from build123d import *

# Parameters (mm, degrees)
ESQUISSE1_W             = 65.4
ESQUISSE1_H             = 56
BOSS_EXTRU_1_DEPTH      = 1.5
CONG_1_R                = 4
ESQUISSE2_R             = 1.4
ENL_V_MAT_EXTRU_1_DEPTH = 1.5
ESQUISSE3_W             = 12.8
ESQUISSE3_H             = 2.56
BOSS_EXTRU_2_DEPTH      = 2.56
ESQUISSE4_W             = 0.6
ESQUISSE4_H             = 13.16
BOSS_EXTRU_3_DEPTH      = 1.58
ENL_V_MAT_EXTRU_2_REACH = 66.012
ESQUISSE5_W             = 5.9
ESQUISSE5_H             = 0.98
BOSS_EXTRU_4_DEPTH      = 2.56
BOSS_EXTRU_5_DEPTH      = 1.8


with BuildPart() as part:
    # Esquisse1 → Boss.-Extru.1 (new body)
    with BuildSketch(Plane(origin=(0, 0, 0), x_dir=(1, 0, 0), z_dir=(0, 1, 0))):
        Rectangle(ESQUISSE1_W, ESQUISSE1_H)
    extrude(amount=BOSS_EXTRU_1_DEPTH)

    # Congé1
    cong_1_edges = [part.edges().sort_by_distance(p)[0] for p in [
        (32.7, 0.75, 28),
        (-32.7, 0.75, 28),
        (-32.7, 0.75, -28),
        (32.7, 0.75, -28),
    ]]
    fillet(cong_1_edges, radius=CONG_1_R)

    # Esquisse2 → Enlèv. mat.-Extru.1 (cut)
    with BuildSketch(Plane(origin=(0, 1.5, 0), x_dir=(1, 0, 0), z_dir=(0, 1, 0))):
        with Locations(Location((-29, 24.5, 0), (0, 0, 270))):
            Circle(ESQUISSE2_R)
        with Locations(Location((-29, -24.5, 0), (0, 0, 270))):
            Circle(ESQUISSE2_R)
        with Locations(Location((29, -24.5, 0), (0, 0, 270))):
            Circle(ESQUISSE2_R)
        with Locations(Location((29, 24.5, 0), (0, 0, 270))):
            Circle(ESQUISSE2_R)
    extrude(amount=-ENL_V_MAT_EXTRU_1_DEPTH, mode=Mode.SUBTRACT)

    # Esquisse3 → Boss.-Extru.2 (add)
    with BuildSketch(Plane(origin=(0, 1.5, 0), x_dir=(1, 0, 0), z_dir=(0, 1, 0))):
        with Locations((-19.3, 19.72)):
            Rectangle(ESQUISSE3_W, ESQUISSE3_H)
    extrude(amount=BOSS_EXTRU_2_DEPTH)

    # Esquisse4 → Boss.-Extru.3 (add)
    with BuildSketch(Plane(origin=(0, 1.5, 0), x_dir=(1, 0, 0), z_dir=(0, 1, 0))):
        with Locations((-24.42, 20.32)):
            Rectangle(ESQUISSE4_W, ESQUISSE4_H)
        with Locations((-21.86, 20.32)):
            Rectangle(ESQUISSE4_W, ESQUISSE4_H)
        with Locations((-19.3, 20.32)):
            Rectangle(ESQUISSE4_W, ESQUISSE4_H)
        with Locations((-16.74, 20.32)):
            Rectangle(ESQUISSE4_W, ESQUISSE4_H)
        with Locations((-14.18, 20.32)):
            Rectangle(ESQUISSE4_W, ESQUISSE4_H)
    extrude(amount=BOSS_EXTRU_3_DEPTH)

    # Enlèv. mat.-Extru.2: up to this face of the body (flat: up to its plane)
    enl_v_mat_extru_2_end = Plane(part.part.faces().sort_by_distance((-13.88, 2.29, -16.09))[0])
    # Esquisse5 → Enlèv. mat.-Extru.2 (cut, up to the picked face)
    with BuildSketch(Plane.ZY.offset(24.72), mode=Mode.PRIVATE) as enl_v_mat_extru_2_sk1:
        with Locations((-23.95, 1.99)):
            Rectangle(ESQUISSE5_W, ESQUISSE5_H)
    enl_v_mat_extru_2_tool1 = split(extrude(enl_v_mat_extru_2_sk1.sketch, amount=-ENL_V_MAT_EXTRU_2_REACH, mode=Mode.PRIVATE), bisect_by=enl_v_mat_extru_2_end, keep=Keep.BOTH, mode=Mode.PRIVATE)
    # Esquisse5 → Enlèv. mat.-Extru.2 (cut, up to the picked face)
    with BuildSketch(Plane.ZY.offset(24.72), mode=Mode.PRIVATE) as enl_v_mat_extru_2_sk2:
        with BuildLine():
            Line((-17.9329542, 3.08), (-15.267871538, 2.100055504))
            Line((-15.267871538, 2.100055504), (-13.74, 2.100055504))
            ThreePointArc((-13.74, 2.100055504), (-13.106146425, 2.552094428), (-13.327063257, 3.298623259))
            Line((-13.327063257, 3.298623259), (-17.9329542, 3.47707173))
            Line((-17.9329542, 3.47707173), (-17.9329542, 3.08))
        make_face()
    enl_v_mat_extru_2_tool2 = split(extrude(enl_v_mat_extru_2_sk2.sketch, amount=-ENL_V_MAT_EXTRU_2_REACH, mode=Mode.PRIVATE), bisect_by=enl_v_mat_extru_2_end, keep=Keep.BOTH, mode=Mode.PRIVATE)
    # Esquisse5 → Enlèv. mat.-Extru.2 (cut, up to the picked face)
    with BuildSketch(Plane.ZY.offset(24.72), mode=Mode.PRIVATE) as enl_v_mat_extru_2_sk3:
        Polygon((-18.44, 2.48), (-18.039767565, 2.48), (-15.374533954, 1.5), (-18.44, 1.5), align=None)
    enl_v_mat_extru_2_tool3 = split(extrude(enl_v_mat_extru_2_sk3.sketch, amount=-ENL_V_MAT_EXTRU_2_REACH, mode=Mode.PRIVATE), bisect_by=enl_v_mat_extru_2_end, keep=Keep.BOTH, mode=Mode.PRIVATE)
    add(enl_v_mat_extru_2_tool1.solids().sort_by(Axis((-24.72, 1.99, -23.95), (1, 0, 0)))[0], mode=Mode.SUBTRACT)
    add(enl_v_mat_extru_2_tool2.solids().sort_by(Axis((-24.72, 2.834984, -15.224036), (1, 0, 0)))[0], mode=Mode.SUBTRACT)
    add(enl_v_mat_extru_2_tool3.solids().sort_by(Axis((-24.72, 1.864391, -17.402771), (1, 0, 0)))[0], mode=Mode.SUBTRACT)

    # Esquisse6 → Boss.-Extru.4 (add)
    with BuildSketch(Plane(origin=(0, 1.5, 0), x_dir=(1, 0, 0), z_dir=(0, 1, 0))):
        Polygon((-31.5, 10.45), (-32.7, 10.45), (-32.7, -10.45), (-31.5, -10.45), (-31.5, -9.8), (-27.1, -9.8), (-27.1, 9.8), (-31.5, 9.8), align=None)
    extrude(amount=BOSS_EXTRU_4_DEPTH)

    # Esquisse7 → Boss.-Extru.5 (add)
    with BuildSketch(Plane(origin=(0, 1.5, 0), x_dir=(1, 0, 0), z_dir=(0, 1, 0))):
        Polygon((-0.5, -18.6), (6.8, -18.6), (6.8, -21.2), (7.7, -21.2), (7.7, -22), (-1.4, -22), (-1.4, -21.2), (-0.5, -21.2), align=None)
    extrude(amount=BOSS_EXTRU_5_DEPTH)


solid = part.part
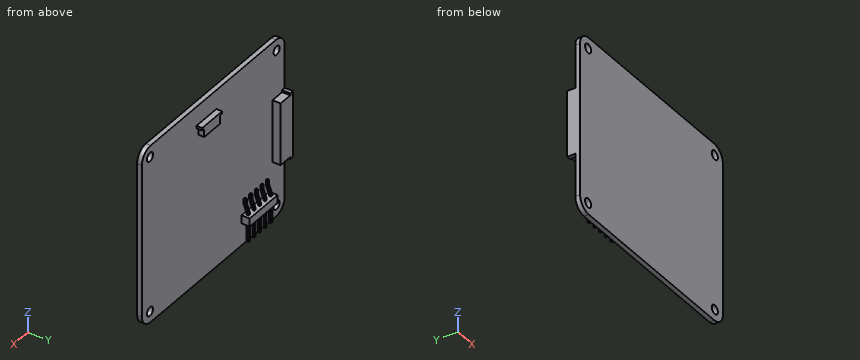
Here's how the part is built. I have some questions about the finished solid (model axes, mm). Round coordinates to 2 decimals unless told otherwise and drop trailing zeros. Write each loop counter-clockwise with the first axis right and the second up, starting at its lowest first coordinate (ties: lowest second). Pieces come first, ordered by that corner, then holes.
1. Suppose I cut it at A-A (z = -22). List the corners of the cut face in (x, y) for me, and give its area (3 significant figures).
2. Suppose I cut it at C-C (x = 23.5). List the corners of the cut face in (y, z) for me.
3. Will these pins go through, and if not, where does the flat tip stop? pin 1 Ø2.5 at (x, z) = (1.5, 20.5) entering from +Y; pin 2 Ø1.5 at (x, z) = (-22.5, 16.5) entering from -Y; pin 3 Ø1.3 at (x, y) = (-29, 3) entering from -Z; pin 4 Ø0.7 at (y, z) = (3, -10) entering from +X.
4. Suppose I cut it at B-B (z = 7.5). List the corners of the cut face in (x, y) for me, and give its area (3 significant figures).
5. I need wall thicknesses on L1, parallel to X at y = 0.3, z = -24.5; L2, parallel to Z at x = -1, y = 2.55; L3, parallel to Y at x = -4, z = -13. Which ranges of each line are inside material? Lowest first, please.
Answer sheet:
1. outline: (-32.7, 0) - (32.7, 0) - (32.7, 1.5) - (-32.7, 1.5) - close; (-24.72, 2.48) - (-24.12, 2.48) - (-24.12, 3.08) - (-24.72, 3.08) - close; (-22.16, 2.48) - (-21.56, 2.48) - (-21.56, 3.08) - (-22.16, 3.08) - close; (-19.6, 2.48) - (-19, 2.48) - (-19, 3.08) - (-19.6, 3.08) - close; (-17.04, 2.48) - (-16.44, 2.48) - (-16.44, 3.08) - (-17.04, 3.08) - close; (-14.48, 2.48) - (-13.88, 2.48) - (-13.88, 3.08) - (-14.48, 3.08) - close
1. area: 99.9 mm2
2. outline: (0, -28) - (1.5, -28) - (1.5, 28) - (0, 28) - close
3. pin 1: stops at y = 3.3
3. pin 2: stops at y = 0
3. pin 3: stops at z = -9.8
3. pin 4: stops at x = -27.1
4. outline: (-32.7, 0) - (32.7, 0) - (32.7, 1.5) - (-27.1, 1.5) - (-27.1, 4.06) - (-32.7, 4.06) - close
4. area: 112 mm2
5. L1: x = -32.67 to -30.4, -27.6 to 27.6, 30.4 to 32.67
5. L2: z = 21.2 to 22
5. L3: y = 0 to 1.5
